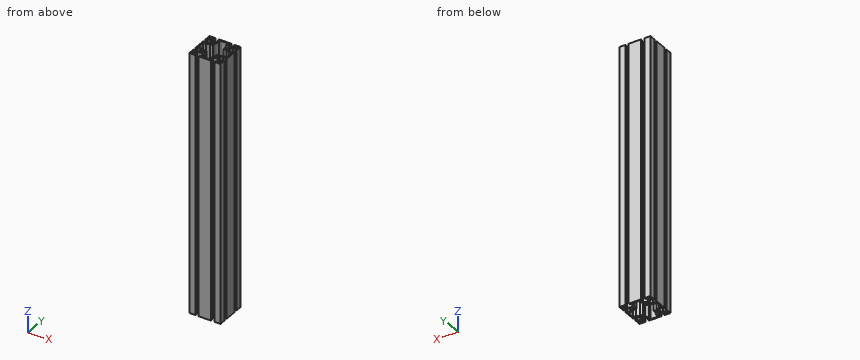
```python
from build123d import *

# Parameters (mm, degrees)
F0_R     = 3
F0_R_2   = 2.5
F1_DEPTH = 500
F2_R     = 2
F3_R     = 7


# Not quite as in the source:
# - a feature names something its author has since deleted; it is built from what else it names


with BuildPart() as f1:
    # F0 (on Top) → F1 (new body)
    with BuildSketch(Plane.XY):
        with BuildLine():
            Line((18.15, -30), (30, -30))
            Line((30, -30), (30, -18.15))
            Line((30, -18.15), (27.5, -18.15))
            Line((27.5, -18.15), (27.5, -20.15))
            Line((27.5, -20.15), (21.5477069044, -20.15))
            ThreePointArc((21.5477069044, -20.15), (19.5, -15), (21.5477069044, -9.85))
            Line((21.5477069044, -9.85), (27.5, -9.85))
            Line((27.5, -9.85), (27.5, -11.85))
            Line((27.5, -11.85), (30, -11.85))
            Line((30, -11.85), (30, 11.85))
            Line((30, 11.85), (27.5, 11.85))
            Line((27.5, 11.85), (27.5, 9.85))
            Line((27.5, 9.85), (21.5477069044, 9.85))
            ThreePointArc((21.5477069044, 9.85), (19.5, 15), (21.5477069044, 20.15))
            Line((21.5477069044, 20.15), (27.5, 20.15))
            Line((27.5, 20.15), (27.5, 18.15))
            Line((27.5, 18.15), (30, 18.15))
            Line((30, 18.15), (30, 30))
            Line((30, 30), (18.15, 30))
            Line((18.15, 30), (18.15, 27.5))
            Line((18.15, 27.5), (20.15, 27.5))
            Line((20.15, 27.5), (20.15, 21.5477069044))
            ThreePointArc((20.15, 21.5477069044), (15, 19.5), (9.85, 21.5477069044))
            Line((9.85, 21.5477069044), (9.85, 27.5))
            Line((9.85, 27.5), (11.85, 27.5))
            Line((11.85, 27.5), (11.85, 30))
            Line((11.85, 30), (-11.85, 30))
            Line((-11.85, 30), (-11.85, 27.5))
            Line((-11.85, 27.5), (-9.85, 27.5))
            Line((-9.85, 27.5), (-9.85, 21.5477069044))
            ThreePointArc((-9.85, 21.5477069044), (-15, 19.5), (-20.15, 21.5477069044))
            Line((-20.15, 21.5477069044), (-20.15, 27.5))
            Line((-20.15, 27.5), (-18.15, 27.5))
            Line((-18.15, 27.5), (-18.15, 30))
            Line((-18.15, 30), (-30, 30))
            Line((-30, 30), (-30, 18.15))
            Line((-30, 18.15), (-27.5, 18.15))
            Line((-27.5, 18.15), (-27.5, 20.15))
            Line((-27.5, 20.15), (-21.5477069044, 20.15))
            ThreePointArc((-21.5477069044, 20.15), (-19.5, 15), (-21.5477069044, 9.85))
            Line((-21.5477069044, 9.85), (-27.5, 9.85))
            Line((-27.5, 9.85), (-27.5, 11.85))
            Line((-27.5, 11.85), (-30, 11.85))
            Line((-30, 11.85), (-30, -11.85))
            Line((-30, -11.85), (-27.5, -11.85))
            Line((-27.5, -11.85), (-27.5, -9.85))
            Line((-27.5, -9.85), (-21.5477069044, -9.85))
            ThreePointArc((-21.5477069044, -9.85), (-19.5, -15), (-21.5477069044, -20.15))
            Line((-21.5477069044, -20.15), (-27.5, -20.15))
            Line((-27.5, -20.15), (-27.5, -18.15))
            Line((-27.5, -18.15), (-30, -18.15))
            Line((-30, -18.15), (-30, -30))
            Line((-30, -30), (-18.15, -30))
            Line((-18.15, -30), (-18.15, -27.5))
            Line((-18.15, -27.5), (-20.15, -27.5))
            Line((-20.15, -27.5), (-20.15, -21.5477069044))
            ThreePointArc((-20.15, -21.5477069044), (-15, -19.5), (-9.85, -21.5477069044))
            Line((-9.85, -21.5477069044), (-9.85, -27.5))
            Line((-9.85, -27.5), (-11.85, -27.5))
            Line((-11.85, -27.5), (-11.85, -30))
            Line((-11.85, -30), (11.85, -30))
            Line((11.85, -30), (11.85, -27.5))
            Line((11.85, -27.5), (9.85, -27.5))
            Line((9.85, -27.5), (9.85, -21.5477069044))
            ThreePointArc((9.85, -21.5477069044), (15, -19.5), (20.15, -21.5477069044))
            Line((20.15, -21.5477069044), (20.15, -27.5))
            Line((20.15, -27.5), (18.15, -27.5))
            Line((18.15, -27.5), (18.15, -30))
        make_face()
        with Locations((-25, -25)):
            Circle(F0_R, mode=Mode.SUBTRACT)
        with Locations((-15, -15)):
            Circle(F0_R_2, mode=Mode.SUBTRACT)
        with Locations((25, -25)):
            Circle(F0_R, mode=Mode.SUBTRACT)
        with Locations((15, -15)):
            Circle(F0_R_2, mode=Mode.SUBTRACT)
        with Locations((-25, 25)):
            Circle(F0_R, mode=Mode.SUBTRACT)
        with Locations((-15, 15)):
            Circle(F0_R_2, mode=Mode.SUBTRACT)
        Polygon((-7, 22), (-7, 27.5), (0, 27.5), (7, 27.5), (7, 22), (10, 16), (10, 10), (16, 10), (22, 7), (27.5, 7), (27.5, 0), (27.5, -7), (22, -7), (16, -10), (10, -10), (10, -16), (7, -22), (7, -27.5), (0, -27.5), (-7, -27.5), (-7, -22), (-10, -16), (-10, -10), (-16, -10), (-22, -7), (-27.5, -7), (-27.5, 0), (-27.5, 7), (-22, 7), (-16, 10), (-10, 10), (-10, 16), align=None, mode=Mode.SUBTRACT)
        with Locations((15, 15)):
            Circle(F0_R_2, mode=Mode.SUBTRACT)
        with Locations((25, 25)):
            Circle(F0_R, mode=Mode.SUBTRACT)
    extrude(amount=F1_DEPTH)

    # F2
    f2_edges = [f1.edges().sort_by_distance(p)[0] for p in [
        (-7, 27.5, 250),
        (7, 27.5, 250),
    ]]
    fillet(f2_edges, radius=F2_R)

    # F3
    f3_edges = [f1.edges().sort_by_distance(p)[0] for p in [
        (-10, 16, 250),
        (10, 16, 250),
    ]]
    fillet(f3_edges, radius=F3_R)


solid = f1.part
```
Can you work these out from the model? Positions are in its coordinate system, mm. Coordinates: 2 decimals unless noted, no trailing zeros. Answer as CSV lines item,"result".
Item 1: Please list where these lines run through material, in increasing order: line 1 along Y through (x, z) = (25, 151); line 2 along Y through (x, z) = (14.5, 180); line 3 along Y through (x, z) = (15, 325).
Geometry results:
line 1,"y = -30 to -28, -22 to -20.15, -9.85 to -7, 7 to 9.85, 20.15 to 22, 28 to 30"
line 2,"y = -19.52 to -17.45, -12.55 to -10, 10 to 12.55, 17.45 to 19.52"
line 3,"y = -19.5 to -17.5, -12.5 to -10, 10 to 12.5, 17.5 to 19.5"
Item 2: Imagine slicing it at A-A on z = 284. State how many separate pieces and enclosed holes the cut face has, plus the area to 3 significant figures.
Geometry results:
separate pieces,"1"
enclosed holes,"9"
area,"1,080 mm2"
Item 3: I'm going to push flat-ended pins straight in: P1, Ø8, axis at x = -17.5, z = 140, coming from the +Y side; P2, Ø1.8, axis at x = 13.5, z = 343, coming from the -Y side; P3, Ø1, axis at y = 15, z = 406.5, coming from the +X side; P4, Ø1.5, axis at x = -16.5, z = 223.5, coming from the +Y side. Where does each tip first touch, or does it pass through?
Geometry results:
P1,"stops at y = 30"
P2,"stops at y = -19.89"
P3,"stops at x = 19.52"
P4,"stops at y = 19.85"
